CAD build for the part. Positions are in the model's coordinates, mm. A direction names the side the tool comes from. Give positions to 0.01 mm unless a question says otherwise; leave off trailing zeros. Write each loop counter-clockwise with the first axis right and the second up, starting at its lowest first coordinate (ties: lowest second). Pieces come first, ordered by that corner, then holes. Notation, with made-up numbers: (-33, -3.5) -> (11, -3.5) arc R17 ccw to (11, 13.5) -> close; hole circle Ø8 at (31, 76.5). An arc over 180 degrees is marked (long way). Use one line per item in the form item = value. Start each with the question number.
from build123d import *

# Parameters (mm, degrees)
SKETCH_W        = 10
SKETCH_H        = 10
PAD_DEPTH       = 5
POCKET_DEPTH    = 3.5
POCKET001_DEPTH = 5.5
POCKET002_DEPTH = 0.25


with BuildPart() as part:
    # Sketch → Pad (new body)
    with BuildSketch(Plane.XY):
        with Locations((5, 5)):
            Rectangle(SKETCH_W, SKETCH_H)
    extrude(amount=PAD_DEPTH)

    # Sketch001 (on Face1 of Pad) → Pocket (cut)
    with BuildSketch(Plane.XZ):
        Polygon((0, 3.9), (0.5, 3.4), (3.5, 3.4), (3.5, 1.6), (0.5, 1.6), (0, 1.1), (-0.843027, 1.1), (-0.843027, 3.9), align=None)
        Polygon((10.955688, 3.9), (10, 3.9), (9.5, 3.4), (6.5, 3.4), (6.5, 1.6), (9.5, 1.6), (10, 1.1), (10.955688, 1.1), align=None)
    extrude(amount=-POCKET_DEPTH, mode=Mode.SUBTRACT)

    # Sketch002 (on Face16 of Pocket) → Pocket001 (cut)
    with BuildSketch(Plane(origin=(0, 10, 0), x_dir=(-1, 0, 0), z_dir=(0, 1, 0))):
        Polygon((-11.13075, 3.9), (-10, 3.9), (-9.5, 3.4), (-6.5, 3.4), (-6.5, 1.6), (-9.5, 1.6), (-10, 1.1), (-11.181449, 1.1), (-11.181449, 3.860271), align=None)
        Polygon((-3.5, 3.4), (-0.5, 3.4), (0, 3.9), (0.82411, 3.9), (0.98968, 1.1), (0, 1.1), (-0.5, 1.6), (-3.5, 1.6), align=None)
    extrude(amount=-POCKET001_DEPTH, mode=Mode.SUBTRACT)

    # Sketch003 (on Face2 of Pocket001) → Pocket002 (cut)
    with BuildSketch(Plane(origin=(0, 0, 0), x_dir=(1, 0, 0), z_dir=(0, 0, -1))):
        Polygon((-0.717832, -0.309342), (-0.717832, -1.992022), (0.739412, -1.150682), align=None)
    extrude(amount=-POCKET002_DEPTH, mode=Mode.SUBTRACT)


solid = part.part
1) Cut at C-C (y = 9.75). Give the cut face in (x, z), and give its area (3 significant figures).
2) Two-plate mould, pull along Z, no slides. Class faces 1 (the face through (2, 7, 1.6)), 2 (the face through (5, 5, 0)), 3 (the face through (5, 10, 2)), 4 (the face through (5, 5, 5)): released by +Z, released by -Z, zero draft, split by the parting line, or undercut.
3) Wall check: line 1 along Z through (x, y) = (2.75, 5.5); line 2 along X through (y, z) = (3, 1.8); line 3 along Y through (x, z) = (9.25, 2.6). Give the ranges that are in metal, low to high. Write a range as from..to.
4) 3-axis set-ups, long thin cutter, end or side, ignore diameter. For faces 5 (the face through (8, 7, 1.6)), 6 (the face through (8, 3.5, 3)), 7 (the face through (2, 4.5, 3)), 8 (the face through (2, 2, 3.4)): which of +Z, -Z, +X, -X, +Y, -Y reach the whole face in a straight line?
5) Pin check, flat tips, straight feed: pin 1 (0.5 mm diameter, centred on y = 2.5, z = 3, fed in from +X); pin 2 (0.9 mm diameter, centred on y = 2, z = 2, fed in from -X); pin 3 (0.8 mm diameter, centred on x = 8.5, z = 2.5, fed in from +Y). Stop position of each tip, or through.
6) Cut at B-B (x = 2.75). Give the cut face in (y, z).
7) Cut at A-A (z = 1.4). Give the cut face in (x, y).
Final values:
q1.outline = (0, 0) -> (10, 0) -> (10, 1.1) -> (9.5, 1.6) -> (6.5, 1.6) -> (6.5, 3.4) -> (9.5, 3.4) -> (10, 3.9) -> (10, 5) -> (0, 5) -> (0, 3.9) -> (0.5, 3.4) -> (3.5, 3.4) -> (3.5, 1.6) -> (0.5, 1.6) -> (0, 1.1) -> close
q1.area = 36.9 mm^2
q2.face_1 = undercut
q2.face_2 = released by -Z
q2.face_3 = zero draft
q2.face_4 = released by +Z
q3.line_1 = 0..1.6, 3.4..5
q3.line_2 = 3.5..6.5
q3.line_3 = 3.5..4.5
q4.face_5 = +X, +Y
q4.face_6 = +X, -Y
q4.face_7 = -X, +Y
q4.face_8 = -X, -Y
q5.pin_1 = 6.5
q5.pin_2 = 0.45
q5.pin_3 = 4.5
q6.outline = (0, 0) -> (10, 0) -> (10, 1.6) -> (4.5, 1.6) -> (4.5, 3.4) -> (10, 3.4) -> (10, 5) -> (0, 5) -> (0, 3.4) -> (3.5, 3.4) -> (3.5, 1.6) -> (0, 1.6) -> close
q7.outline = (0, 3.5) -> (0.3, 3.5) -> (0.3, 0) -> (9.7, 0) -> (9.7, 3.5) -> (10, 3.5) -> (10, 4.5) -> (9.7, 4.5) -> (9.7, 10) -> (0.3, 10) -> (0.3, 4.5) -> (0, 4.5) -> close
